Geometry check sheet. Reference: the model listing, model coordinates, mm. Face numbers are marked on the shaded views. A direction names the side the tool comes from. Round coordinates to 2 decimals unless told otherwise and drop trailing zeros. Order: outer loops, then holes, each group sorted by start corner. A loop starts at its lowest first (then second) coordinate and runs counter-clockwise, first axis right, second up.
(1) Cross-section at C-C on z = 18.5. Enter the section's corners in (x, y).
(2) Set-up check for the marked faces 1 and 2: record each of +Z, -Z, +X, -X, +Y, -Y from which the full face is reachable in a straight line by a thin tool's end or side.
(3) Gauge pin test, flat ends, axial feed: P1, Ø15, axis at x = -38, z = 28.5, coming from the +Y side; P2, Ø17, axis at x = 1, z = 14.5, coming from the -Y side; P3, Ø2, axis at y = 19.5, z = 46.5, coming from the +X side. Record the tip position at first contact, or that the pin passes through.
(4) Thickness scan on L1, parallel to X at y = 7, z = 12.5; L2, parallel to X at y = 15, z = 53.5; L3, parallel to Y at x = -9.5, z = 45. Record the ranges inside material, lowest first.
(5) Draft check along X on the marked faces 3, 4, 5 and 6. Enter one of: pulls with the +X half, pulls with the -X half, needs draft (parallel to the pull), parting line crosses it, or undercut.
(6) Cross-section at A-A on y = -16. Enter the section's corners in (x, z).
(7) Cross-section at B-B on x = -75. Enter the section's corners in (y, z).
from build123d import *

# Parameters (mm, degrees)
SKETCH045_W  = 300
SKETCH045_H  = 60
PAD007_DEPTH = 250
SKETCH046_W  = 312
SKETCH046_H  = 50
PAD008_DEPTH = 256
SKETCH047_W  = 412
SKETCH047_H  = 612
PAD009_DEPTH = 6


with BuildPart() as body008:
    # Sketch045 → Pad007 (new body, symmetric)
    with BuildSketch(Plane.XZ):
        with Locations((0, 30)):
            Rectangle(SKETCH045_W, SKETCH045_H)
    extrude(amount=PAD007_DEPTH, both=True)


with BuildPart() as cut005:
    # Sketch046 → Pad008 (new body, symmetric)
    with BuildSketch(Plane.XZ):
        with Locations((0, 25)):
            Rectangle(SKETCH046_W, SKETCH046_H)
    extrude(amount=PAD008_DEPTH, both=True)

    # Sketch047 (on Face3 of Pad008) → Pad009 (join)
    with BuildSketch(Plane(origin=(0, 0, 50), x_dir=(-1, 0, 0), z_dir=(0, 0, 1))):
        Rectangle(SKETCH047_W, SKETCH047_H)
    extrude(amount=PAD009_DEPTH)

    # Cut005: cut Body008
    add(body008.part, mode=Mode.SUBTRACT)


solid = cut005.part
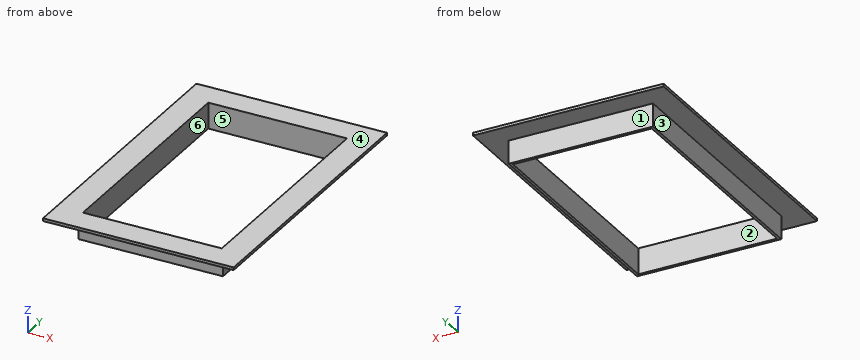
Found:
1. outline: (-156, -256) - (156, -256) - (156, 256) - (-156, 256) - close; hole (-150, -250) - (150, -250) - (150, 250) - (-150, 250) - close
2. face 1: -Z, +X, -X, +Y
2. face 2: +Z, -Z
3. P1: stops at y = 256
3. P2: stops at y = -256
3. P3: stops at x = 156
4. L1: x = -156 to -150, 150 to 156
4. L2: x = -206 to -150, 150 to 206
4. L3: y = -256 to -250, 250 to 256
5. face 3: pulls with the -X half
5. face 4: needs draft
5. face 5: undercut
5. face 6: undercut
6. outline: (-206, 50) - (-156, 50) - (-156, 0) - (-150, 0) - (-150, 56) - (-206, 56) - close; (150, 0) - (156, 0) - (156, 50) - (206, 50) - (206, 56) - (150, 56) - close
7. outline: (-306, 50) - (-256, 50) - (-256, 0) - (-250, 0) - (-250, 56) - (-306, 56) - close; (250, 0) - (256, 0) - (256, 50) - (306, 50) - (306, 56) - (250, 56) - close
